from build123d import *

# Parameters (mm, degrees)
SKETCH1_R               = 28.575
BOSS_EXTRUDE1_DEPTH     = 6.35
F_1_4_20_TAPPED_HOLE1_D = 5.1054
SKETCH5_R               = 11
CUT_EXTRUDE1_DEPTH      = 7.35
F_10_32_TAPPED_HOLE1_D  = 4.0386


with BuildPart() as part:
    # Sketch1 → Boss-Extrude1 (new body)
    with BuildSketch(Plane(origin=(0, 0, 0), x_dir=(1, 0, 0), z_dir=(0, 1, 0))):
        Circle(SKETCH1_R)
    extrude(amount=BOSS_EXTRUDE1_DEPTH)

    # 1/4-20 Tapped Hole1 (through all)
    with Locations(Plane(origin=(0, 6.35, 0), x_dir=(1, 0, 0), z_dir=(0, 1, 0))):
        with Locations((0, 23.8125), (20.622229928, 11.90625), (20.622229928, -11.90625), (0, -23.8125), (-20.622229928, -11.90625), (-20.622229928, 11.90625)):
            Hole(F_1_4_20_TAPPED_HOLE1_D / 2)

    # Sketch5 → Cut-Extrude1 (cut, through all)
    with BuildSketch(Plane(origin=(0, 6.35, 0), x_dir=(1, 0, 0), z_dir=(0, 1, 0))):
        Circle(SKETCH5_R)
    extrude(amount=-CUT_EXTRUDE1_DEPTH, mode=Mode.SUBTRACT)

    # #10-32 Tapped Hole1 (through all)
    with Locations(Plane(origin=(0, 6.35, 0), x_dir=(1, 0, 0), z_dir=(0, 1, 0))):
        with Locations((-8.73125, 15.122968614), (8.73125, 15.122968614), (17.4625, 0), (8.73125, -15.122968614), (-8.73125, -15.122968614), (-17.4625, 0)):
            Hole(F_10_32_TAPPED_HOLE1_D / 2)


solid = part.part
Design review of the part built by this model. Coordinates are the model's own, in mm. Round coordinates to 2 decimals unless told otherwise and drop trailing zeros. Order: outer loops, then holes, each group sorted by start corner. A loop starts at its lowest first (then second) coordinate and runs counter-clockwise, first axis right, second up.
1) Draft analysis for pull direction X (two halves, no side actions). For faces 1 (the cylindrical face through (-28.547, 3.131, -1.256)), 2 (the cylindrical face through (-22.98, 3.13, 12.88)), 3 (the flat face through (0, 0, 12)), state which applies: released by +X, released by -X, zero draft, split by the parting line, or undercut.
The answers:
face 1: split by the parting line
face 2: undercut
face 3: zero draft
2) Consider section D-D (x = -21.5). State the section outline as (y, z) points, plus the area to 3 significant figures.
The answers:
outline: (0, -18.82) - (6.35, -18.82) - (6.35, -14.3) - (0, -14.3) - close; (0, -9.51) - (6.35, -9.51) - (6.35, 9.51) - (0, 9.51) - close; (0, 14.3) - (6.35, 14.3) - (6.35, 18.82) - (0, 18.82) - close
area: 178 mm2
3) Consider section C-C (z = 7). State the section outline as (x, y) points.
The answers:
outline: (-27.7, 0) - (-8.49, 0) - (-8.49, 6.35) - (-27.7, 6.35) - close; (8.49, 0) - (27.7, 0) - (27.7, 6.35) - (8.49, 6.35) - close
4) Consider section B-B (z = 0). State the section outline as (x, y) points (3 decimals).
The answers:
outline: (-28.575, 0) - (-19.482, 0) - (-19.482, 6.35) - (-28.575, 6.35) - close; (-15.443, 0) - (-11, 0) - (-11, 6.35) - (-15.443, 6.35) - close; (11, 0) - (15.443, 0) - (15.443, 6.35) - (11, 6.35) - close; (19.482, 0) - (28.575, 0) - (28.575, 6.35) - (19.482, 6.35) - close
5) Consider section A-A (x = 0). State the section outline as (y, z) points (3 decimals).
The answers:
outline: (0, -28.575) - (6.35, -28.575) - (6.35, -26.365) - (0, -26.365) - close; (0, -21.26) - (6.35, -21.26) - (6.35, -11) - (0, -11) - close; (0, 11) - (6.35, 11) - (6.35, 21.26) - (0, 21.26) - close; (0, 26.365) - (6.35, 26.365) - (6.35, 28.575) - (0, 28.575) - close
6) Clearance check with flat-ended pins moving along their axes: pin 1 Ø3 at (y, z) = (1, 10.5) entering from +X; pin 2 Ø6 at (x, z) = (20.62, 11.91) entering from +Y; pin 3 Ø3 at (x, y) = (14.5, 2) entering from -Z; pin 4 Ø2 at (x, y) = (-17.5, 1) entering from +Z. State where each tip first meets the part, or that it passes through.
The answers:
pin 1: stops at x = 27.12
pin 2: stops at y = 6.35
pin 3: stops at z = -25.45
pin 4: stops at z = 23.33
7) For L1, parallel to Z at x = 0, y = 2.5 (3 decimals); L2, parallel to Z at x = 7.5, y = 3; L3, parallel to X at y = 1, z = -1.5, list the stretches that pass through material, from the lowest coordinate up.
The answers:
L1: z = -28.575 to -26.365, -21.26 to -11, 11 to 21.26, 26.365 to 28.575
L2: z = -27.57 to -16.72, -13.52 to -8.05, 8.05 to 13.52, 16.72 to 27.57
L3: x = -28.54 to -18.81, -16.11 to -10.9, 10.9 to 16.11, 18.81 to 28.54
